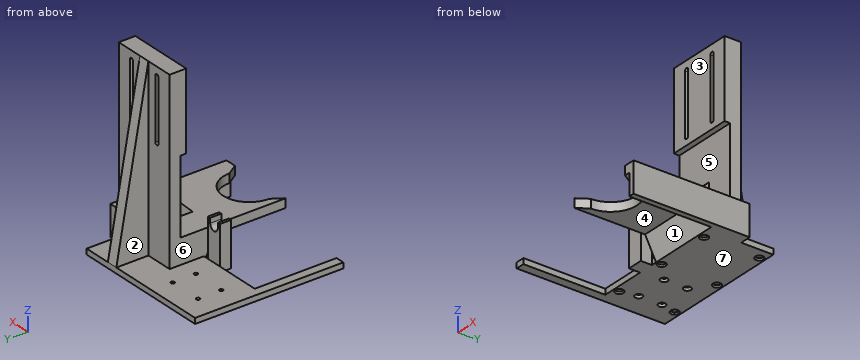
from build123d import *

# Parameters (mm, degrees)
SKETCH_1_W                   = 120
SKETCH_1_H                   = 60
EXTRUDE_1_DEPTH              = 5
SKETCH_3_W                   = 60
SKETCH_3_H                   = 8
EXTRUDE_3_DEPTH              = 60
EXTRUDE_6_DEPTH              = 10
SKETCH_11_R                  = 1.6
CUT_EXTRUDE_3_DEPTH          = 124.668912828
SKETCH_12_R                  = 1.6
CUT_EXTRUDE_4_DEPTH          = 134.603892159
SKETCH_18_R                  = 3.75
CUT_EXTRUDE_7_DEPTH          = 2
SKETCH_20_W                  = 60
SKETCH_20_H                  = 90
EXTRUDE_8_DEPTH              = 8
SKETCH_22_W                  = 60
SKETCH_22_H                  = 50
EXTRUDE_9_DEPTH              = 5
CUT_EXTRUDE_8_DEPTH          = 191.131533418
CUT_EXTRUDE_8_DEPTH_BACK     = 191.131533418
SKETCH_23_W                  = 60
SKETCH_23_H                  = 10
EXTRUDE_10_DEPTH             = 160
CUT_EXTRUDE_9_DEPTH          = 190.660222503
SKETCH_25_W                  = 150
SKETCH_25_H                  = 13
CUT_EXTRUDE_10_DEPTH         = 193.937813816
SKETCH_26_W                  = 60
SKETCH_26_H                  = 8
EXTRUDE_11_DEPTH             = 85
SKETCH_27_R                  = 23.5
CUT_EXTRUDE_11_DEPTH         = 181.364214854
EXTRUDE_12_DEPTH             = 8
SKETCH_29_W                  = 60
SKETCH_29_H                  = 70
EXTRUDE_13_DEPTH             = 5
CUT_EXTRUDE_12_DEPTH         = 207.276513447
HOLE_WIZARD_M3_1_D           = 3.2
HOLE_WIZARD_M3_1_CSINK_D     = 6.6
HOLE_WIZARD_M3_1_CSINK_ANGLE = 90
SKETCH_33_W                  = 14.5
SKETCH_33_H                  = 21
EXTRUDE_14_DEPTH             = 60
EXTRUDE_15_DEPTH             = 60
EXTRUDE_18_DEPTH             = 5
EXTRUDE_19_DEPTH             = 5
SKETCH_38_W                  = 10
SKETCH_38_H                  = 105
EXTRUDE_20_DEPTH             = 8
SKETCH_40_W                  = 10
SKETCH_40_H                  = 19.5
EXTRUDE_21_DEPTH             = 105
CUT_EXTRUDE_13_DEPTH         = 5
SKETCH_42_W                  = 8
SKETCH_42_H                  = 134
EXTRUDE_22_DEPTH             = 5
EXTRUDE_17_DEPTH             = 5


with BuildPart() as part:
    # 草图1 → 凸台-拉伸1 (new body)
    with BuildSketch(Plane.XY):
        with Locations((-25, 50)):
            Rectangle(SKETCH_1_W, SKETCH_1_H)
    extrude(amount=EXTRUDE_1_DEPTH)

    # 草图3 → 凸台-拉伸3 (add)
    with BuildSketch(Plane.XY.offset(5)):
        with Locations((5, 76)):
            Rectangle(SKETCH_3_W, SKETCH_3_H)
    extrude(amount=EXTRUDE_3_DEPTH)

    # 草图9 → 凸台-拉伸6 (add)
    with BuildSketch(Plane.XZ.offset(-20)):
        with BuildLine():
            Line((-32.5, 0), (-41.5, 0))
            Line((-41.5, 0), (-44, 0))
            Line((-44, 0), (-44, 40))
            Line((-44, 40), (-41.5, 40))
            Line((-41.5, 40), (-41.5, 35.5))
            ThreePointArc((-41.5, 35.5), (-37, 31), (-32.5, 35.5))
            Line((-32.5, 35.5), (-32.5, 40))
            Line((-32.5, 40), (-30, 40))
            Line((-30, 40), (-30, 0))
            Line((-30, 0), (-32.5, 0))
        make_face()
    extrude(amount=EXTRUDE_6_DEPTH)

    # 草图11 → 切除-拉伸3 (cut, through all)
    with BuildSketch(Plane(origin=(0, 72, 0), x_dir=(-1, 0, 0), z_dir=(0, -1, 0))):
        with Locations(Location((-20, -52.088110118, 0), (0, 0, 90))):
            Circle(SKETCH_11_R)
        with Locations(Location((10, -28.088110118, 0), (0, 0, 90))):
            Circle(SKETCH_11_R)
        with Locations(Location((-20, -28.088110118, 0), (0, 0, 90))):
            Circle(SKETCH_11_R)
        with Locations(Location((10, -52.088110118, 0), (0, 0, 90))):
            Circle(SKETCH_11_R)
    extrude(amount=-CUT_EXTRUDE_3_DEPTH, mode=Mode.SUBTRACT)

    # 草图12 → 切除-拉伸4 (cut, through all)
    with BuildSketch(Plane(origin=(0, 0, 0), x_dir=(-1, 0, 0), z_dir=(0, 0, -1))):
        with Locations((42, 40.25)):
            Circle(SKETCH_12_R)
        with Locations((42, 61.25)):
            Circle(SKETCH_12_R)
        with Locations((72, 40.25)):
            Circle(SKETCH_12_R)
        with Locations((72, 61.25)):
            Circle(SKETCH_12_R)
    extrude(amount=-CUT_EXTRUDE_4_DEPTH, mode=Mode.SUBTRACT)

    # 草图18 → 切除-拉伸7 (cut)
    with BuildSketch(Plane(origin=(0, 0, 0), x_dir=(-1, 0, 0), z_dir=(0, 0, -1))):
        with Locations((75, 75)):
            Circle(SKETCH_18_R)
        with Locations((25, 75)):
            Circle(SKETCH_18_R)
        with Locations((-25, 75)):
            Circle(SKETCH_18_R)
        with Locations((-25, 25)):
            Circle(SKETCH_18_R)
        with Locations((25, 25)):
            Circle(SKETCH_18_R)
        with Locations((75, 25)):
            Circle(SKETCH_18_R)
    extrude(amount=-CUT_EXTRUDE_7_DEPTH, mode=Mode.SUBTRACT)

    # 草图20 → 凸台-拉伸8 (add)
    with BuildSketch(Plane(origin=(0, 80, 0), x_dir=(1, 0, 0), z_dir=(0, 1, 0))):
        with Locations((5, -110)):
            Rectangle(SKETCH_20_W, SKETCH_20_H)
    extrude(amount=-EXTRUDE_8_DEPTH)

    # 草图22 → 凸台-拉伸9 (add)
    with BuildSketch(Plane.XZ.offset(-72)):
        with Locations((5, 130)):
            Rectangle(SKETCH_22_W, SKETCH_22_H)
    extrude(amount=EXTRUDE_9_DEPTH)

    # 草图21 → 切除-拉伸8 (cut, two sides: drawn at the far end of the back side and taken through both)
    with BuildSketch(Plane(origin=(0, 80, 0), x_dir=(1, 0, 0), z_dir=(0, 1, 0)).offset(-CUT_EXTRUDE_8_DEPTH_BACK)):
        with BuildLine():
            Line((21.75, -115), (21.75, -145))
            ThreePointArc((21.75, -145), (20, -146.75), (18.25, -145))
            Line((18.25, -145), (18.25, -115))
            ThreePointArc((18.25, -115), (20, -113.25), (21.75, -115))
        make_face()
        with BuildLine():
            Line((-11.75, -115), (-11.75, -145))
            ThreePointArc((-11.75, -145), (-10, -146.75), (-8.25, -145))
            Line((-8.25, -145), (-8.25, -115))
            ThreePointArc((-8.25, -115), (-10, -113.25), (-11.75, -115))
        make_face()
    extrude(amount=CUT_EXTRUDE_8_DEPTH + CUT_EXTRUDE_8_DEPTH_BACK, mode=Mode.SUBTRACT)

    # 草图23 → 凸台-拉伸10 (add)
    with BuildSketch(Plane.XY.offset(5)):
        with Locations((5, 46)):
            Rectangle(SKETCH_23_W, SKETCH_23_H)
    extrude(amount=EXTRUDE_10_DEPTH)

    # 草图24 → 切除-拉伸9 (cut, through all)
    with BuildSketch(Plane.XZ.offset(-41)):
        with BuildLine():
            Line((-8.25, 157), (-8.25, 102))
            ThreePointArc((-8.25, 102), (-10, 100.25), (-11.75, 102))
            Line((-11.75, 102), (-11.75, 157))
            ThreePointArc((-11.75, 157), (-10, 158.75), (-8.25, 157))
        make_face()
        with BuildLine():
            Line((18.25, 157), (18.25, 102))
            ThreePointArc((18.25, 102), (20, 100.25), (21.75, 102))
            Line((21.75, 102), (21.75, 157))
            ThreePointArc((21.75, 157), (20, 158.75), (18.25, 157))
        make_face()
    extrude(amount=-CUT_EXTRUDE_9_DEPTH, mode=Mode.SUBTRACT)

    # 草图25 → 切除-拉伸10 (cut, through all)
    with BuildSketch(Plane.ZY.offset(25)):
        with Locations((80, 73.5)):
            Rectangle(SKETCH_25_W, SKETCH_25_H)
    extrude(amount=-CUT_EXTRUDE_10_DEPTH, mode=Mode.SUBTRACT)

    # 草图26 → 凸台-拉伸11 (add)
    with BuildSketch(Plane.XZ.offset(-41)):
        with Locations((5, 23.5)):
            Rectangle(SKETCH_26_W, SKETCH_26_H)
    extrude(amount=EXTRUDE_11_DEPTH)

    # 草图27 → 切除-拉伸11 (cut, through all)
    with BuildSketch(Plane.XY.offset(27.5)):
        with Locations((5, -44)):
            Circle(SKETCH_27_R)
    extrude(amount=-CUT_EXTRUDE_11_DEPTH, mode=Mode.SUBTRACT)

    # 草图28 → 凸台-拉伸12 (add)
    with BuildSketch(Plane.XY.offset(27.5)):
        Polygon((35, -44), (35, -54), (28.5, -44), align=None)
        Polygon((-25, -44), (-25, -54), (-18.5, -44), align=None)
    extrude(amount=-EXTRUDE_12_DEPTH)

    # 草图29 → 凸台-拉伸13 (add)
    with BuildSketch(Plane.XZ.offset(-41)):
        with Locations((5, 130)):
            Rectangle(SKETCH_29_W, SKETCH_29_H)
    extrude(amount=EXTRUDE_13_DEPTH)

    # 草图30 → 切除-拉伸12 (cut, through all)
    with BuildSketch(Plane.XZ.offset(-36)):
        with BuildLine():
            Line((18.25, 102), (18.25, 157))
            ThreePointArc((18.25, 157), (20, 158.75), (21.75, 157))
            Line((21.75, 157), (21.75, 102))
            ThreePointArc((21.75, 102), (20, 100.25), (18.25, 102))
        make_face()
        with BuildLine():
            Line((-8.25, 102), (-8.25, 157))
            ThreePointArc((-8.25, 157), (-10, 158.75), (-11.75, 157))
            Line((-11.75, 157), (-11.75, 102))
            ThreePointArc((-11.75, 102), (-10, 100.25), (-8.25, 102))
        make_face()
    extrude(amount=-CUT_EXTRUDE_12_DEPTH, mode=Mode.SUBTRACT)

    # M3 十字槽沉头木螺钉的锥形沉头孔1 (through all)
    with Locations(Plane(origin=(0, 0, 0), x_dir=(-1, 0, 0), z_dir=(0, 0, -1))):
        with Locations((42, 61.25), (72, 61.25), (72, 40.25), (42, 40.25)):
            CounterSinkHole(HOLE_WIZARD_M3_1_D / 2, HOLE_WIZARD_M3_1_CSINK_D / 2, counter_sink_angle=HOLE_WIZARD_M3_1_CSINK_ANGLE)

    # 草图33 → 凸台-拉伸14 (add)
    with BuildSketch(Plane(origin=(35, 0, 0), x_dir=(0, 0, -1), z_dir=(1, 0, 0))):
        with Locations((-12.25, 30.5)):
            Rectangle(SKETCH_33_W, SKETCH_33_H)
    extrude(amount=-EXTRUDE_14_DEPTH)

    # 草图34 → 凸台-拉伸15 (add)
    with BuildSketch(Plane(origin=(35, 0, 0), x_dir=(0, 0, -1), z_dir=(1, 0, 0))):
        Polygon((-19.5, 10), (0, 20), (-19.5, 20), align=None)
    extrude(amount=-EXTRUDE_15_DEPTH)

    # 草图35 → 凸台-拉伸18 (add, symmetric)
    with BuildSketch(Plane(origin=(5, 0, 0), x_dir=(0, 0, -1), z_dir=(1, 0, 0))):
        Polygon((-57.5, 41), (-27.5, 11), (-27.5, 41), align=None)
    extrude(amount=EXTRUDE_18_DEPTH, both=True)

    # 草图37 → 凸台-拉伸19 (add, symmetric)
    with BuildSketch(Plane(origin=(5, 0, 0), x_dir=(0, 0, -1), z_dir=(1, 0, 0))):
        Polygon((-5, 80), (-165, 51), (-5, 51), align=None)
    extrude(amount=EXTRUDE_19_DEPTH, both=True)

    # 草图38 → 凸台-拉伸20 (add)
    with BuildSketch(Plane.XY.offset(27.5)):
        with Locations((40, -1.5)):
            Rectangle(SKETCH_38_W, SKETCH_38_H)
    extrude(amount=-EXTRUDE_20_DEPTH)

    # 草图40 → 凸台-拉伸21 (add)
    with BuildSketch(Plane.XZ.offset(54)):
        with Locations((40, 9.75)):
            Rectangle(SKETCH_40_W, SKETCH_40_H)
    extrude(amount=-EXTRUDE_21_DEPTH)

    # 草图41 → 切除-拉伸13 (cut)
    with BuildSketch(Plane.ZY.offset(-35)):
        Polygon((0, 20), (19.5, 10), (19.5, -54), (0, -54), align=None)
    extrude(amount=-CUT_EXTRUDE_13_DEPTH, mode=Mode.SUBTRACT)

    # 草图42 → 凸台-拉伸22 (add)
    with BuildSketch(Plane.XY.offset(5)):
        with Locations((-89, 13)):
            Rectangle(SKETCH_42_W, SKETCH_42_H)
    extrude(amount=-EXTRUDE_22_DEPTH)

    # 草图36 → 凸台-拉伸17 (add, symmetric)
    with BuildSketch(Plane(origin=(5, 0, 0), x_dir=(0, 0, -1), z_dir=(1, 0, 0))):
        Polygon((-5, 80), (-165, 51), (-5, 51), align=None)
    extrude(amount=EXTRUDE_17_DEPTH, both=True)


solid = part.part
Geometry check sheet. Reference: the model listing, model coordinates, mm. Face numbers are marked on the shaded views. A direction names the side the tool comes from. Give positions to 0.01 mm unless a question says otherwise; leave off trailing zeros. Loops run counter-clockwise (first coordinate to the right, second up) from the corner with the lowest first, then second, coordinate; pieces in that order, holes last. Notation, with made-up numbers: M 7.25,35 L 39.25,35 A19 cw 39.25,69 Z; hole C 31.5,15.5 d1. An arc over 180 degrees is marked long. Answer as a JSON object with one key per item and string values. Group by question number.
Item 1: Sectioned sample at B-B on y = 16. Record the boundary of the cut face in (x, z).
Item 2: Sectioned sample at D-D on y = 48.5. Record the boundary of the cut face in (x, z).
Item 3: Mould release check, pull along Z, two halves, no side actions. Record for the marked faces 5, 6 and 7: pulls with the +Z half, pulls with the -Z half, needs draft (parallel to the pull), parting line crosses it, or undercut.
Item 4: Material ranges on L1, parallel to X at y = 61, z = 2; L2, parallel to X at y = 40.25, z = 3.6; L3, parallel to Y at x = -6, z = 72.5, recorded low to high.
Item 5: Sectioned sample at A-A on y = -12. Record the boundary of the cut face in (x, z).
Item 6: Access from +Z, -Z, +X, -X, +Y, -Y to the whole of each face (thin tool, end or side, straight path). Record for the marked faces 1, 2, 3 and 4.
Item 7: Gauge pin test, flat ends, axial feed: pin 1 (2 mm diameter, centred on x = 8.5, y = 33.5, fed in from +Z); pin 2 (1.5 mm diameter, centred on y = 42, z = 35, fed in from -X); pin 3 (20 mm diameter, centred on x = 21.5, y = 65.5, fed in from +Z). Record the tip position at first contact, or that the pin passes through.
Item 8: Sectioned sample at C-C on z = 152. Record the boundary of the cut face in (x, y).
Findings below:
{
 "1": {"outline": "M -93,0 L -85,0 L -85,5 L -93,5 Z; M -44,0 L -30,0 L -30,40 L -32.5,40 L -32.5,35.5 A4.5 cw -41.5,35.5 L -41.5,40 L -44,40 Z; M -25,7.8 L 40,7.8 L 40,0 L 45,0 L 45,27.5 L 10,27.5 L 10,32.5 L 0,32.5 L 0,27.5 L -25,27.5 Z"},
 "2": {"outline": "M -93,0 L 45,0 L 45,27.5 L 35,27.5 L 35,165 L -25,165 L -25,5 L -93,5 Z; hole M -11.75,102 A1.75 ccw -8.25,102 L -8.25,157 A1.75 ccw -11.75,157 Z; hole M 18.25,102 A1.75 ccw 21.75,102 L 21.75,157 A1.75 ccw 18.25,157 Z"},
 "3": {"face 5": "undercut", "face 6": "needs draft", "face 7": "pulls with the -Z half"},
 "4": {"L1": "-93 to -73.58, -70.42 to -43.58, -40.42 to 35", "L2": "-93 to -73.6, -70.4 to -43.6, -40.4 to 45", "L3": "41 to 51"},
 "5": {"outline": "M -93,0 L -85,0 L -85,5 L -93,5 Z; M -25,19.5 L 40,19.5 L 40,0 L 45,0 L 45,27.5 L -25,27.5 Z"},
 "6": {"face 1": "-Z, -Y", "face 2": "+Z, -X, +Y", "face 3": "+Z, +X, -X, -Y", "face 4": "-Z, -X, -Y"},
 "7": {"pin 1": "z = 51", "pin 2": "x = -25", "pin 3": "z = 5"},
 "8": {"outline": "M -25,36 L -11.75,36 L -11.75,51 L -25,51 Z; M -8.25,36 L 18.25,36 L 18.25,51 L 10,51 L 10,53.36 L 0,53.36 L 0,51 L -8.25,51 Z; M 21.75,36 L 35,36 L 35,51 L 21.75,51 Z"}
}
